from build123d import *

# Parameters (mm, degrees)
SKIZZE1_W                       = 50
SKIZZE1_H                       = 114
AUFSATZ_LINEAR_AUSTRAGEN1_DEPTH = 60
SKIZZE2_W                       = 46
SKIZZE2_H                       = 110
SCHNITT_LINEAR_AUSTRAGEN1_DEPTH = 58
SKIZZE3_R                       = 2
AUFSATZ_LINEAR_AUSTRAGEN2_DEPTH = 15.2
SKIZZE4_R                       = 0.5
SCHNITT_LINEAR_AUSTRAGEN2_DEPTH = 5
SCHNITT_LINEAR_AUSTRAGEN3_REACH = 123.846
SKIZZE5_W                       = 15.5
SKIZZE5_H                       = 20.2
SKIZZE6_W                       = 15.5
SKIZZE6_H                       = 2
AUFSATZ_LINEAR_AUSTRAGEN3_DEPTH = 1
SCHNITT_LINEAR_AUSTRAGEN4_REACH = 123.846
SKIZZE7_W                       = 40
SKIZZE7_H                       = 3.1
FASE1_SIZE                      = 1.5
SKIZZE8_W                       = 10
SKIZZE8_H                       = 6.5
SCHNITT_LINEAR_AUSTRAGEN5_DEPTH = 3
SCHNITT_LINEAR_AUSTRAGEN6_REACH = 133.996
SKIZZE9_R                       = 3.8
SCHNITT_LINEAR_AUSTRAGEN7_REACH = 133.996
SKIZZE10_W                      = 9
SKIZZE10_H                      = 3.5


with BuildPart() as part:
    # Skizze1 → Aufsatz-Linear austragen1 (new body)
    with BuildSketch(Plane(origin=(0, 0, 0), x_dir=(1, 0, 0), z_dir=(0, 1, 0))):
        with Locations((3.757679181, -46.225255973)):
            Rectangle(SKIZZE1_W, SKIZZE1_H)
    extrude(amount=AUFSATZ_LINEAR_AUSTRAGEN1_DEPTH)

    # Skizze2 → Schnitt-Linear austragen1 (cut)
    with BuildSketch(Plane(origin=(0, 60, 0), x_dir=(1, 0, 0), z_dir=(0, 1, 0))):
        with Locations((3.757679181, -46.225255973)):
            Rectangle(SKIZZE2_W, SKIZZE2_H)
    extrude(amount=-SCHNITT_LINEAR_AUSTRAGEN1_DEPTH, mode=Mode.SUBTRACT)

    # Skizze3 → Aufsatz-Linear austragen2 (add)
    with BuildSketch(Plane(origin=(0, 2, 0), x_dir=(1, 0, 0), z_dir=(0, 1, 0))):
        with Locations(Location((-11.242320819, -24.225255973, 0), (0, 0, 90))):
            Circle(SKIZZE3_R)
        with Locations(Location((18.757679181, -24.225255973, 0), (0, 0, 90))):
            Circle(SKIZZE3_R)
        with Locations(Location((18.757679181, -96.225255973, 0), (0, 0, 90))):
            Circle(SKIZZE3_R)
        with Locations(Location((-11.242320819, -96.225255973, 0), (0, 0, 90))):
            Circle(SKIZZE3_R)
    extrude(amount=AUFSATZ_LINEAR_AUSTRAGEN2_DEPTH)

    # Skizze4 → Schnitt-Linear austragen2 (cut)
    with BuildSketch(Plane(origin=(0, 17.2, 0), x_dir=(1, 0, 0), z_dir=(0, 1, 0))):
        with Locations(Location((-11.242320819, -24.225255973, 0), (0, 0, 270))):
            Circle(SKIZZE4_R)
        with Locations(Location((18.757679181, -24.225255973, 0), (0, 0, 270))):
            Circle(SKIZZE4_R)
        with Locations(Location((18.757679181, -96.225255973, 0), (0, 0, 270))):
            Circle(SKIZZE4_R)
        with Locations(Location((-11.242320819, -96.225255973, 0), (0, 0, 270))):
            Circle(SKIZZE4_R)
    extrude(amount=-SCHNITT_LINEAR_AUSTRAGEN2_DEPTH, mode=Mode.SUBTRACT)

    # Skizze5 → Schnitt-Linear austragen3 (cut, up to next)
    with BuildSketch(Plane(origin=(0, 2, 0), x_dir=(1, 0, 0), z_dir=(0, 1, 0)), mode=Mode.PRIVATE) as schnitt_linear_austragen3_sk1:
        with Locations((3.757679181, -17.825255973)):
            Rectangle(SKIZZE5_W, SKIZZE5_H)
    schnitt_linear_austragen3_tool1 = extrude(schnitt_linear_austragen3_sk1.sketch, amount=-SCHNITT_LINEAR_AUSTRAGEN3_REACH, mode=Mode.PRIVATE) & part.part
    add(schnitt_linear_austragen3_tool1.solids().sort_by_distance((3.757679, 2, 17.825256))[0], mode=Mode.SUBTRACT)

    # Skizze6 → Aufsatz-Linear austragen3 (add)
    with BuildSketch(Plane(origin=(0, 2, 0), x_dir=(1, 0, 0), z_dir=(0, 1, 0))):
        with Locations((3.757679181, -28.925255973)):
            Rectangle(SKIZZE6_W, SKIZZE6_H)
    extrude(amount=AUFSATZ_LINEAR_AUSTRAGEN3_DEPTH)

    # Skizze7 → Schnitt-Linear austragen4 (cut, up to next)
    with BuildSketch(Plane(origin=(0, 2, 0), x_dir=(1, 0, 0), z_dir=(0, 1, 0)), mode=Mode.PRIVATE) as schnitt_linear_austragen4_sk1:
        with Locations((3.757679181, -34.775255973)):
            Rectangle(SKIZZE7_W, SKIZZE7_H)
    schnitt_linear_austragen4_tool1 = extrude(schnitt_linear_austragen4_sk1.sketch, amount=-SCHNITT_LINEAR_AUSTRAGEN4_REACH, mode=Mode.PRIVATE) & part.part
    # Skizze7 → Schnitt-Linear austragen4 (cut, up to next)
    with BuildSketch(Plane(origin=(0, 2, 0), x_dir=(1, 0, 0), z_dir=(0, 1, 0)), mode=Mode.PRIVATE) as schnitt_linear_austragen4_sk2:
        with Locations((3.757679181, -38.875255973)):
            Rectangle(SKIZZE7_W, SKIZZE7_H)
    schnitt_linear_austragen4_tool2 = extrude(schnitt_linear_austragen4_sk2.sketch, amount=-SCHNITT_LINEAR_AUSTRAGEN4_REACH, mode=Mode.PRIVATE) & part.part
    # Skizze7 → Schnitt-Linear austragen4 (cut, up to next)
    with BuildSketch(Plane(origin=(0, 2, 0), x_dir=(1, 0, 0), z_dir=(0, 1, 0)), mode=Mode.PRIVATE) as schnitt_linear_austragen4_sk3:
        with Locations((3.757679181, -42.975255973)):
            Rectangle(SKIZZE7_W, SKIZZE7_H)
    schnitt_linear_austragen4_tool3 = extrude(schnitt_linear_austragen4_sk3.sketch, amount=-SCHNITT_LINEAR_AUSTRAGEN4_REACH, mode=Mode.PRIVATE) & part.part
    # Skizze7 → Schnitt-Linear austragen4 (cut, up to next)
    with BuildSketch(Plane(origin=(0, 2, 0), x_dir=(1, 0, 0), z_dir=(0, 1, 0)), mode=Mode.PRIVATE) as schnitt_linear_austragen4_sk4:
        with Locations((3.757679181, -47.075255973)):
            Rectangle(SKIZZE7_W, SKIZZE7_H)
    schnitt_linear_austragen4_tool4 = extrude(schnitt_linear_austragen4_sk4.sketch, amount=-SCHNITT_LINEAR_AUSTRAGEN4_REACH, mode=Mode.PRIVATE) & part.part
    # Skizze7 → Schnitt-Linear austragen4 (cut, up to next)
    with BuildSketch(Plane(origin=(0, 2, 0), x_dir=(1, 0, 0), z_dir=(0, 1, 0)), mode=Mode.PRIVATE) as schnitt_linear_austragen4_sk5:
        with Locations((3.757679181, -51.175255973)):
            Rectangle(SKIZZE7_W, SKIZZE7_H)
    schnitt_linear_austragen4_tool5 = extrude(schnitt_linear_austragen4_sk5.sketch, amount=-SCHNITT_LINEAR_AUSTRAGEN4_REACH, mode=Mode.PRIVATE) & part.part
    # Skizze7 → Schnitt-Linear austragen4 (cut, up to next)
    with BuildSketch(Plane(origin=(0, 2, 0), x_dir=(1, 0, 0), z_dir=(0, 1, 0)), mode=Mode.PRIVATE) as schnitt_linear_austragen4_sk6:
        with Locations((3.757679181, -55.275255973)):
            Rectangle(SKIZZE7_W, SKIZZE7_H)
    schnitt_linear_austragen4_tool6 = extrude(schnitt_linear_austragen4_sk6.sketch, amount=-SCHNITT_LINEAR_AUSTRAGEN4_REACH, mode=Mode.PRIVATE) & part.part
    add(schnitt_linear_austragen4_tool1.solids().sort_by_distance((3.757679, 2, 34.775256))[0], mode=Mode.SUBTRACT)
    add(schnitt_linear_austragen4_tool2.solids().sort_by_distance((3.757679, 2, 38.875256))[0], mode=Mode.SUBTRACT)
    add(schnitt_linear_austragen4_tool3.solids().sort_by_distance((3.757679, 2, 42.975256))[0], mode=Mode.SUBTRACT)
    add(schnitt_linear_austragen4_tool4.solids().sort_by_distance((3.757679, 2, 47.075256))[0], mode=Mode.SUBTRACT)
    add(schnitt_linear_austragen4_tool5.solids().sort_by_distance((3.757679, 2, 51.175256))[0], mode=Mode.SUBTRACT)
    add(schnitt_linear_austragen4_tool6.solids().sort_by_distance((3.757679, 2, 55.275256))[0], mode=Mode.SUBTRACT)

    # Fase1
    fase1_edges = [part.edges().sort_by_distance(p)[0] for p in [
        (-16.242320819, 1, 36.325255973),
        (-16.242320819, 1, 33.225255973),
        (23.757679181, 1, 33.225255973),
        (23.757679181, 1, 36.325255973),
        (-16.242320819, 1, 37.325255973),
        (23.757679181, 1, 37.325255973),
        (23.757679181, 1, 40.425255973),
        (-16.242320819, 1, 40.425255973),
        (-16.242320819, 1, 41.425255973),
        (23.757679181, 1, 41.425255973),
        (23.757679181, 1, 44.525255973),
        (-16.242320819, 1, 44.525255973),
        (-16.242320819, 1, 45.525255973),
        (23.757679181, 1, 45.525255973),
        (23.757679181, 1, 48.625255973),
        (-16.242320819, 1, 48.625255973),
        (-16.242320819, 1, 49.625255973),
        (23.757679181, 1, 49.625255973),
        (23.757679181, 1, 52.725255973),
        (-16.242320819, 1, 52.725255973),
        (-16.242320819, 1, 53.725255973),
        (23.757679181, 1, 53.725255973),
        (23.757679181, 1, 56.825255973),
        (-16.242320819, 1, 56.825255973),
    ]]
    chamfer(fase1_edges, length=FASE1_SIZE)

    # Skizze8 → Schnitt-Linear austragen5 (cut)
    with BuildSketch(Plane(origin=(28.757679181, 0, 0), x_dir=(0, 0, -1), z_dir=(1, 0, 0))):
        with Locations((-55.225255973, 3.25)):
            Rectangle(SKIZZE8_W, SKIZZE8_H)
    extrude(amount=-SCHNITT_LINEAR_AUSTRAGEN5_DEPTH, mode=Mode.SUBTRACT)

    # Skizze9 → Schnitt-Linear austragen6 (cut, up to next)
    with BuildSketch(Plane(origin=(0, 0, -10.774744027), x_dir=(-1, 0, 0), z_dir=(0, 0, -1)), mode=Mode.PRIVATE) as schnitt_linear_austragen6_sk1:
        with BuildLine():
            Line((7.442320819, 60), (7.442320819, 50))
            ThreePointArc((7.442320819, 50), (11.242320819, 53.8), (15.042320819, 50))
            Line((15.042320819, 50), (15.042320819, 60))
            Line((15.042320819, 60), (7.442320819, 60))
        make_face()
    schnitt_linear_austragen6_tool1 = extrude(schnitt_linear_austragen6_sk1.sketch, amount=-SCHNITT_LINEAR_AUSTRAGEN6_REACH, mode=Mode.PRIVATE) & part.part
    # Skizze9 → Schnitt-Linear austragen6 (cut, up to next)
    with BuildSketch(Plane(origin=(0, 0, -10.774744027), x_dir=(-1, 0, 0), z_dir=(0, 0, -1)), mode=Mode.PRIVATE) as schnitt_linear_austragen6_sk2:
        with Locations((11.242320819, 50)):
            Circle(SKIZZE9_R)
    schnitt_linear_austragen6_tool2 = extrude(schnitt_linear_austragen6_sk2.sketch, amount=-SCHNITT_LINEAR_AUSTRAGEN6_REACH, mode=Mode.PRIVATE) & part.part
    add(schnitt_linear_austragen6_tool1.solids().sort_by_distance((-11.242321, 56.440988, -10.774744))[0], mode=Mode.SUBTRACT)
    add(schnitt_linear_austragen6_tool2.solids().sort_by_distance((-11.242321, 50, -10.774744))[0], mode=Mode.SUBTRACT)

    # Skizze10 → Schnitt-Linear austragen7 (cut, up to next)
    with BuildSketch(Plane.XY.offset(103.225255973), mode=Mode.PRIVATE) as schnitt_linear_austragen7_sk1:
        with Locations((12.007679181, 56.25)):
            Rectangle(SKIZZE10_W, SKIZZE10_H)
    schnitt_linear_austragen7_tool1 = extrude(schnitt_linear_austragen7_sk1.sketch, amount=-SCHNITT_LINEAR_AUSTRAGEN7_REACH, mode=Mode.PRIVATE) & part.part
    add(schnitt_linear_austragen7_tool1.solids().sort_by_distance((12.007679, 56.25, 103.225256))[0], mode=Mode.SUBTRACT)


solid = part.part
Geometry: final body of the model. Coordinates: model frame, mm. A direction names the side the tool comes from. Give positions to 0.01 mm unless a question says otherwise; leave off trailing zeros. Order: outer loops, then holes, each group sorted by start corner. A loop starts at its lowest first (then second) coordinate and runs counter-clockwise, first axis right, second up. Notation, with made-up numbers: (-31, 45.5) -> (5, 45.5) arc R25 cw to (5, 64.5) -> close; hole circle Ø9 at (72, 49). An arc over 180 degrees is marked (long way). Put each result on its own line as item: value.
Q1. Draft query along Z for faces 1 (the face through (4, 1, 27.925)), 2 (the face through (28.758, 30, 47)), 3 (the face through (3, 30, 103.225)). Return one class per face: released by +Z, released by -Z, zero draft, split by the parting line, or undercut.
Here are the results:
face 1: undercut
face 2: zero draft
face 3: released by +Z
Q2. Section B-B, the plane z = 65. Return loops of the section in (x, y), then the cut area to 3 significant figures.
Here are the results:
outline: (-21.24, 0) -> (28.76, 0) -> (28.76, 60) -> (26.76, 60) -> (26.76, 2) -> (-19.24, 2) -> (-19.24, 60) -> (-21.24, 60) -> close
area: 332 mm^2
Q3. Pin query (flat end, axial travel): pin 1 (12 mm diameter, centred on x = 17.5, z = 41.5, fed in from +Y); pin 2 (1.6 mm diameter, centred on y = 1, z = 55.5, fed in from +X); pin 3 (0.8 mm diameter, centred on x = -11.5, z = 96.5, fed in from +Y). Return the tip coordinate at first contact, or that it passes through.
Here are the results:
pin 1: stops at y = 2
pin 2: stops at x = 25.76
pin 3: stops at y = 17.2
Q4. Section C-C, the plane x = 4. Count the separate pieces of the cut face and the enclosed holes in it, then the cut area to 3 significant figures.
Here are the results:
separate pieces: 8
enclosed holes: 0
area: 384 mm^2
Q5. Material intervals for L1, parallel to Z at x = 11, y = 17.5; L2, parallel to X at y = 17, z = 32; L3, parallel to Z at x = 17, y = 9, sorted ascending.
Here are the results:
L1: z = -10.77 to -8.77, 101.23 to 103.23
L2: x = -21.24 to -19.24, 26.76 to 28.76
L3: z = -10.77 to -8.77, 23.27 to 25.18, 95.27 to 97.18, 101.23 to 103.23
Q6. Section A-A, the plane y = 26. Return loops of the section in (x, z), then the cut area to 3 significant figures.
Here are the results:
outline: (-21.24, -10.77) -> (28.76, -10.77) -> (28.76, 103.23) -> (-21.24, 103.23) -> close; hole (-19.24, -8.77) -> (26.76, -8.77) -> (26.76, 101.23) -> (-19.24, 101.23) -> close
area: 640 mm^2
Q7. Reachability of faces 4 (the face through (3, 0, 45)), 5 (the face through (-9.3, 9.5, 24.7)) from +Z, -Z, +X, -X, +Y, -Y: full face, straight path, thin tool, end or side. Return the list, or none.
Here are the results:
face 4: +Z, -Z, +X, -X, -Y
face 5: +Y
